Could you check a few things on this model? Use its own coordinates, in mm. A direction names the side the tool comes from. Round coordinates to 2 decimals unless told otherwise and drop trailing zeros. Loops run counter-clockwise (first coordinate to the right, second up) from the corner with the lowest first, then second, coordinate; pieces in that order, holes last. Notation, with made-up numbers: (85, 89.5) -> (138, 89.5) arc R16 cw to (138, 111.5) -> close; hole circle Ø7 at (82, 57.5). An arc over 180 degrees is marked (long way). Write each question's results on one line, items separated by ' | '.
from build123d import *

# Parameters (mm, degrees)
F0_W     = 31.75
F0_H     = 50.8
F1_DEPTH = 12.7
F2_W     = 12.7
F2_H     = 50.8
F3_DEPTH = 19.05
F5_DEPTH = 25.4
F6_W     = 12.7
F6_H     = 19.05
F7_DEPTH = 19.05
F9_DEPTH = 25.4


with BuildPart() as f1:
    # F0 (on Top) → F1 (new body)
    with BuildSketch(Plane.XY):
        with Locations((15.875, 25.4)):
            Rectangle(F0_W, F0_H)
    extrude(amount=F1_DEPTH)

    # F2 (on face) → F3 (join)
    with BuildSketch(Plane.XY.offset(12.7)):
        with Locations((6.35, 25.4)):
            Rectangle(F2_W, F2_H)
    extrude(amount=F3_DEPTH)

    # F4 (on face) → F5 (cut)
    with BuildSketch(Plane.YZ.offset(12.7)):
        Polygon((50.8, 12.7), (50.8, 31.75), (38.1, 31.75), align=None)
    extrude(amount=-F5_DEPTH, mode=Mode.SUBTRACT)

    # F6 (on face) → F7 (join)
    with BuildSketch(Plane.YZ.offset(12.7)):
        with Locations((22.702408, 22.225)):
            Rectangle(F6_W, F6_H)
    extrude(amount=F7_DEPTH)

    # F8 (on face) → F9 (cut)
    with BuildSketch(Plane.XZ.offset(-16.352408)):
        Polygon((31.75, 12.7), (31.75, 31.75), (12.7, 31.75), align=None)
    extrude(amount=-F9_DEPTH, mode=Mode.SUBTRACT)


solid = f1.part
1) For faces 1 (the flat face through (12.7, 8, 22)), 2 (the flat face through (20, 29.052, 20)), 3 (the flat face through (0, 25, 16)), which set-ups out of +Z, -Z, +X, -X, +Y, -Y let a thin tool reach every point of the face, with its end or its side?
Model answer:
face 1: +Z, +X, -Y | face 2: +Z, +X, +Y | face 3: +Z, -Z, -X, +Y, -Y
2) I want a section at D-D, the plane x = 6.5. Write out the boundary of the cut face in (y, z), plus the area to 3 significant figures.
Model answer:
outline: (0, 0) -> (50.8, 0) -> (50.8, 12.7) -> (38.1, 31.75) -> (0, 31.75) -> close | area: 1,490 mm2
3) I'm going to push flat-ended pins straight in: pin 1 (12 mm diameter, centred on y = 14, z = 15.5, fed in from +X); pin 2 (8 mm diameter, centred on x = 24, y = 5, fed in from +Z); pin 3 (1 mm diameter, centred on y = 26.5, z = 24, fed in from +X); pin 4 (5 mm diameter, centred on y = 5, z = 19.5, fed in from +X). Where does each tip first touch, or does it pass through?
Model answer:
pin 1: stops at x = 31.75 | pin 2: stops at z = 12.7 | pin 3: stops at x = 20.95 | pin 4: stops at x = 12.7
4) I want a section at C-C, the plane y = 46.5. Write out the boundary of the cut face in (x, z).
Model answer:
outline: (0, 0) -> (31.75, 0) -> (31.75, 12.7) -> (12.7, 12.7) -> (12.7, 19.15) -> (0, 19.15) -> close
5) I want a section at B-B, the plane z = 20.5. Write out the boundary of the cut face in (x, y), plus the area to 3 significant figures.
Model answer:
outline: (0, 0) -> (12.7, 0) -> (12.7, 16.35) -> (23.95, 16.35) -> (23.95, 29.05) -> (12.7, 29.05) -> (12.7, 45.6) -> (0, 45.6) -> close | area: 722 mm2
6) I want a section at A-A, the plane x = 22. Write out the boundary of the cut face in (y, z), plus the area to 3 significant figures.
Model answer:
outline: (0, 0) -> (50.8, 0) -> (50.8, 12.7) -> (29.05, 12.7) -> (29.05, 22.45) -> (16.35, 22.45) -> (16.35, 12.7) -> (0, 12.7) -> close | area: 769 mm2
7) I need wall thicknesses on line 1 (Y direction, x = 16.5, z = 16.5); line 2 (X direction, y = 8, z = 28). Which ranges of each line are inside material? Lowest first, please.
Model answer:
line 1: y = 16.35 to 29.05 | line 2: x = 0 to 12.7
